Model file for the job. Use its own axes, mm. Face numbers are marked on the shaded views. A direction names the side the tool comes from. Coordinates: 2 decimals unless noted, no trailing zeros. Order: outer loops, then holes, each group sorted by start corner. A loop starts at its lowest first (then second) coordinate and runs counter-clockwise, first axis right, second up. Notation, with made-up numbers: (9, -36) - (48, -36) arc R26 ccw to (48, -22) - close; hole circle Ø11 at (-11.75, 72). An arc over 180 degrees is marked (long way). Put each result on its own line as item: value. Start each with the question number.
```python
from build123d import *

# Parameters (mm, degrees)
EXTRUDE_1_DEPTH     = 6
SKETCH_2_R          = 1.5
CUT_EXTRUDE_1_DEPTH = 16.663731995


with BuildPart() as part:
    # 草圖1 → 填料-伸長1 (new body)
    with BuildSketch(Plane(origin=(0, 0, 0), x_dir=(0, 0, -1), z_dir=(1, 0, 0))):
        Polygon((-12.25, 0), (12.25, 0), (12.25, 2.8), (6.4, 2.8), (6.4, 10.5), (2, 10.5), (2, 2.8), (-2, 2.8), (-2, 10.5), (-6.4, 10.5), (-6.4, 2.8), (-12.25, 2.8), align=None)
    extrude(amount=EXTRUDE_1_DEPTH)

    # 草圖2 → 除料-伸長1 (cut, through all)
    with BuildSketch(Plane(origin=(0, 2.8, 0), x_dir=(1, 0, 0), z_dir=(0, 1, 0))):
        with Locations(Location((3, 9.25, 0), (0, 0, 270))):
            Circle(SKETCH_2_R)
    cut_extrude_1 = extrude(amount=-CUT_EXTRUDE_1_DEPTH, mode=Mode.SUBTRACT)

    # 鏡射1: 除料-伸長1 across plane
    add(cut_extrude_1.mirror(Plane.XY), mode=Mode.SUBTRACT)


solid = part.part
```
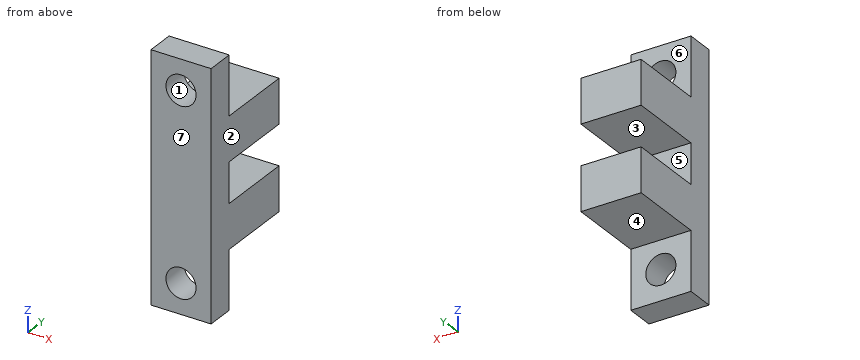
Item 1: Slice it at D-D, the plane x = 3. Give the cut face in (y, z).
Item 2: Slice it at C-C, the plane y = 3.75. Give the cut face in (x, z).
Item 3: Slice it at A-A, the plane x = 1.8. Give the cut face in (y, z).
Item 4: Pull direction X, two halves, no side cores. Call the marked faces 1, 2 and 3: pulls with the +X half, pulls with the -X half, needs draft (parallel to the pull), parting line crosses it, or undercut.
Item 5: Flat gauge pins, fed straight in: pin 1 Ø3 at (x, y) = (4.5, 4.5) entering from -Z; pin 2 Ø1.2 at (x, z) = (3, 0.5) entering from +Y; pin 3 Ø3 at (x, y) = (2, 8) entering from +Z. Where does each tip first touch, or does it go through?
Item 6: Wall check: line 1 along X through (y, z) = (0.6, 9.25); line 2 along Z through (x, y) = (1.6, 3.75); line 3 along Z through (x, y) = (4.35, 1.25). Give the ranges that are in metal, low to high.
Item 7: 3-axis set-ups, long thin cutter, end or side, ignore diameter. For the marked faces 4, 5, 6 and 7: which of +Z, -Z, +X, -X, +Y, -Y reach the whole face in a straight line?
Item 8: Slice it at B-B, the plane z = -9.25. Give the cut face in (x, y).
Here are the results:
1. outline: (0, -12.25) - (2.8, -12.25) - (2.8, -10.75) - (0, -10.75) - close; (0, -7.75) - (2.8, -7.75) - (2.8, -6.4) - (10.5, -6.4) - (10.5, -2) - (2.8, -2) - (2.8, 2) - (10.5, 2) - (10.5, 6.4) - (2.8, 6.4) - (2.8, 7.75) - (0, 7.75) - close; (0, 10.75) - (2.8, 10.75) - (2.8, 12.25) - (0, 12.25) - close
2. outline: (0, -6.4) - (6, -6.4) - (6, -2) - (0, -2) - close; (0, 2) - (6, 2) - (6, 6.4) - (0, 6.4) - close
3. outline: (0, -12.25) - (2.8, -12.25) - (2.8, -10.15) - (0, -10.15) - close; (0, -8.35) - (2.8, -8.35) - (2.8, -6.4) - (10.5, -6.4) - (10.5, -2) - (2.8, -2) - (2.8, 2) - (10.5, 2) - (10.5, 6.4) - (2.8, 6.4) - (2.8, 8.35) - (0, 8.35) - close; (0, 10.15) - (2.8, 10.15) - (2.8, 12.25) - (0, 12.25) - close
4. face 1: undercut
4. face 2: pulls with the +X half
4. face 3: needs draft
5. pin 1: stops at z = -6.4
5. pin 2: stops at y = 2.8
5. pin 3: stops at z = 6.4
6. line 1: x = 0 to 1.5, 4.5 to 6
6. line 2: z = -6.4 to -2, 2 to 6.4
6. line 3: z = -12.25 to -9.9, -8.6 to 8.6, 9.9 to 12.25
7. face 4: -Z, +X, -X, +Y
7. face 5: +X, -X, +Y
7. face 6: +Z, +X, -X, +Y
7. face 7: +Z, -Z, +X, -X, -Y
8. outline: (0, 0) - (1.5, 0) - (1.5, 2.8) - (0, 2.8) - close; (4.5, 0) - (6, 0) - (6, 2.8) - (4.5, 2.8) - close
